```python
from build123d import *

# Parameters (mm, degrees)
SKETCH1_W              = 126
SKETCH1_H              = 126
BOSS_EXTRUDE1_DEPTH    = 5.5
CUT_EXTRUDE5_DEPTH     = 179.275769526
SKETCH8_R              = 10
CUT_EXTRUDE6_DEPTH     = 179.275769526
FILLET1_R              = 5.5
FILLET2_R              = 2.75
SKETCH11_W             = 13
SKETCH11_H             = 13
CUT_EXTRUDE7_DEPTH     = 179.275769526
BOSS_EXTRUDE8_START    = -15
SKETCH18_R             = 2
BOSS_EXTRUDE8_DEPTH    = 10
BOSS_EXTRUDE9_START    = -75
SKETCH18_2_R           = 2
BOSS_EXTRUDE9_DEPTH    = 10
BOSS_EXTRUDE10_DEPTH   = 10
BOSS_EXTRUDE11_DEPTH   = 3
BOSS_EXTRUDE12_DEPTH   = 4.692640137
BOSS_EXTRUDE12_START   = -13
BOSS_EXTRUDE12_2_DEPTH = 14
BOSS_EXTRUDE13_DEPTH   = 4.692640137
BOSS_EXTRUDE13_START   = -127
BOSS_EXTRUDE13_2_DEPTH = 14
CHAMFER1_SIZE          = 2


with BuildPart() as part:
    # Sketch1 → Boss-Extrude1 (new body)
    with BuildSketch(Plane(origin=(0, 0, 0), x_dir=(1, 0, 0), z_dir=(0, 1, 0))):
        with Locations((63, 63)):
            Rectangle(SKETCH1_W, SKETCH1_H)
    extrude(amount=BOSS_EXTRUDE1_DEPTH)

    # Sketch7 → Cut-Extrude5 (cut, through all)
    with BuildSketch(Plane.XY):
        Polygon((0, 0), (0, 5.5), (5.5, 5.5), align=None)
        Polygon((126, 0), (126, 5.5), (120.5, 5.5), align=None)
    cut_extrude5 = extrude(amount=-CUT_EXTRUDE5_DEPTH, mode=Mode.SUBTRACT)

    # Mirror1: Cut-Extrude5 across plane
    add(cut_extrude5.mirror(Plane(origin=(0, 0, 0), x_dir=(-0.7071067811865476, 0, 0.7071067811865476), z_dir=(-0.7071067811865477, 0, -0.7071067811865475))), mode=Mode.SUBTRACT)

    # Sketch8 → Cut-Extrude6 (cut, through all)
    with BuildSketch(Plane(origin=(0, 5.5, 0), x_dir=(1, 0, 0), z_dir=(0, 1, 0))):
        with Locations(Location((63, 63, 0), (0, 0, 270))):
            Circle(SKETCH8_R)
        with BuildLine():
            Line((50.269180349, 54.158267646), (8.5, 12.389087297))
            Line((8.5, 12.389087297), (8.5, 113.610912703))
            Line((8.5, 113.610912703), (50.269180349, 71.841732354))
            ThreePointArc((50.269180349, 71.841732354), (47.5, 63), (50.269180349, 54.158267646))
        make_face()
        with BuildLine():
            Line((54.158267646, 75.730819651), (12.389087297, 117.5))
            Line((12.389087297, 117.5), (113.610912703, 117.5))
            Line((113.610912703, 117.5), (71.841732354, 75.730819651))
            ThreePointArc((71.841732354, 75.730819651), (63, 78.5), (54.158267646, 75.730819651))
        make_face()
        with BuildLine():
            Line((75.730819651, 71.841732354), (117.5, 113.610912703))
            Line((117.5, 113.610912703), (117.5, 12.389087297))
            Line((117.5, 12.389087297), (75.730819651, 54.158267646))
            ThreePointArc((75.730819651, 54.158267646), (78.5, 63), (75.730819651, 71.841732354))
        make_face()
        with BuildLine():
            Line((71.841732354, 50.269180349), (113.610912703, 8.5))
            Line((113.610912703, 8.5), (12.389087297, 8.5))
            Line((12.389087297, 8.5), (54.158267646, 50.269180349))
            ThreePointArc((54.158267646, 50.269180349), (63, 47.5), (71.841732354, 50.269180349))
        make_face()
    extrude(amount=-CUT_EXTRUDE6_DEPTH, mode=Mode.SUBTRACT)

    # Fillet1
    fillet1_edges = [part.edges().sort_by_distance(p)[0] for p in [
        (113.610912703, 2.75, -8.5),
        (12.389087297, 2.75, -8.5),
        (117.5, 2.75, -113.610912703),
        (117.5, 2.75, -12.389087297),
        (12.389087297, 2.75, -117.5),
        (113.610912703, 2.75, -117.5),
        (8.5, 2.75, -12.389087297),
        (8.5, 2.75, -113.610912703),
    ]]
    fillet(fillet1_edges, radius=FILLET1_R)

    # Fillet2
    fillet2_edges = [part.edges().sort_by_distance(p)[0] for p in [
        (54.158267646, 2.75, -50.269180349),
        (71.841732354, 2.75, -50.269180349),
        (75.730819651, 2.75, -54.158267646),
        (75.730819651, 2.75, -71.841732354),
        (71.841732354, 2.75, -75.730819651),
        (54.158267646, 2.75, -75.730819651),
        (50.269180349, 2.75, -71.841732354),
        (50.269180349, 2.75, -54.158267646),
    ]]
    fillet(fillet2_edges, radius=FILLET2_R)

    # Sketch11 → Cut-Extrude7 (cut, through all)
    with BuildSketch(Plane(origin=(0, 5.5, 0), x_dir=(1, 0, 0), z_dir=(0, 1, 0))):
        with Locations((6.5, 119.5)):
            Rectangle(SKETCH11_W, SKETCH11_H)
        with Locations((119.5, 119.5)):
            Rectangle(SKETCH11_W, SKETCH11_H)
        with Locations((119.5, 6.5)):
            Rectangle(SKETCH11_W, SKETCH11_H)
        with Locations((6.5, 6.5)):
            Rectangle(SKETCH11_W, SKETCH11_H)
    extrude(amount=-CUT_EXTRUDE7_DEPTH, mode=Mode.SUBTRACT)

    # Sketch18 → Boss-Extrude8 (add)
    with BuildSketch(Plane(origin=(0, 0, -113), x_dir=(-1, 0, 0), z_dir=(0, 0, -1)).offset(BOSS_EXTRUDE8_START)):
        with BuildLine():
            Line((-6.5, 0), (0.5, 0))
            ThreePointArc((0.5, 0), (8.363703305, 1.03527618), (1.035898385, -2))
            Line((1.035898385, -2), (-6.5, -2))
            Line((-6.5, -2), (-6.5, 0))
        make_face()
        with Locations((4.5, 0)):
            Circle(SKETCH18_R, mode=Mode.SUBTRACT)
    extrude(amount=-BOSS_EXTRUDE8_DEPTH)

    # Sketch18<2> → Boss-Extrude9 (add)
    with BuildSketch(Plane(origin=(0, 0, -113), x_dir=(-1, 0, 0), z_dir=(0, 0, -1)).offset(BOSS_EXTRUDE9_START)):
        with BuildLine():
            Line((-6.5, 0), (0.5, 0))
            ThreePointArc((0.5, 0), (8.363703305, 1.03527618), (1.035898385, -2))
            Line((1.035898385, -2), (-6.5, -2))
            Line((-6.5, -2), (-6.5, 0))
        make_face()
        with Locations((4.5, 0)):
            Circle(SKETCH18_2_R, mode=Mode.SUBTRACT)
    extrude(amount=-BOSS_EXTRUDE9_DEPTH)

    # Sketch19 → Boss-Extrude10 (add)
    with BuildSketch(Plane.XZ):
        Polygon((126, -113), (113, -113), (113, -126), (110, -126), (110, -110), (126, -110), align=None)
        Polygon((126, -16), (126, -13), (113, -13), (113, 0), (110, 0), (110, -16), align=None)
    extrude(amount=BOSS_EXTRUDE10_DEPTH)

    # Sketch20 → Boss-Extrude11 (add)
    with BuildSketch(Plane.XZ.offset(10)):
        Polygon((110, -16), (126, -16), (126, -13), (128, -13), (128, 2), (113, 2), (113, 0), (110, 0), align=None)
        Polygon((126, -110), (126, -113), (128, -113), (128, -128), (113, -128), (113, -126), (110, -126), (110, -110), align=None)
    extrude(amount=BOSS_EXTRUDE11_DEPTH)

    # Boss-Extrude12: read off the stored shape, not the designer's step
    # Boss-Extrude12 outline → Boss-Extrude12 (add)
    with BuildSketch(Plane.ZY.offset(-13)):
        Polygon((-13, 5.5), (-13, 0), (0, 0), (-5.5, 5.5), align=None)
    extrude(amount=BOSS_EXTRUDE12_DEPTH)

    # Boss-Extrude12 2 outline → Boss-Extrude12 2 (cut)
    with BuildSketch(Plane.XY.offset(BOSS_EXTRUDE12_START)):
        with BuildLine():
            Line((8.307359863, 0), (11.819098493, 0))
            ThreePointArc((11.819098493, 0), (10.365939115, 2.943279669), (8.307359863, 5.5))
            Line((8.307359863, 5.5), (8.307359863, 0))
        make_face()
    extrude(amount=BOSS_EXTRUDE12_2_DEPTH, mode=Mode.SUBTRACT)

    # Boss-Extrude13: read off the stored shape, not the designer's step
    # Boss-Extrude13 outline → Boss-Extrude13 (add)
    with BuildSketch(Plane.ZY.offset(-13)):
        Polygon((-120.5, 5.5), (-126, 0), (-113, 0), (-113, 5.5), align=None)
    extrude(amount=BOSS_EXTRUDE13_DEPTH)

    # Boss-Extrude13 2 outline → Boss-Extrude13 2 (cut)
    with BuildSketch(Plane.XY.offset(BOSS_EXTRUDE13_START)):
        with BuildLine():
            ThreePointArc((11.819098492, 0), (10.365939114, 2.943279669), (8.307359863, 5.5))
            Line((8.307359863, 5.5), (8.307359863, 0))
            Line((8.307359863, 0), (11.819098492, 0))
        make_face()
    extrude(amount=BOSS_EXTRUDE13_2_DEPTH, mode=Mode.SUBTRACT)

    # Chamfer1
    chamfer1_edges = [part.edges().sort_by_distance(p)[0] for p in [
        (6.5, 0, -93),
        (6.5, 0, -33),
    ]]
    chamfer(chamfer1_edges, length=CHAMFER1_SIZE - 0.0001)  # a hair under: the kernel refuses the full size


solid = part.part
```
Verification items for the finished model (mm, model axes). A direction names the side the tool comes from. Give positions to 0.01 mm unless a question says otherwise; leave off trailing zeros. Loops run counter-clockwise (first coordinate to the right, second up) from the corner with the lowest first, then second, coordinate; pieces in that order, holes last.
1. Go/stop test with flat-tipped pins: pin 1 Ø0.6 at (y, z) = (-12, -127) entering from -X; pin 2 Ø8.5 at (x, z) = (3, -33.5) entering from -Y; pin 3 Ø4 at (x, z) = (2, -95.5) entering from -Y. Record where each tip stops, or that it passes through.
2. Set-up check for faces 5 (the cylindrical face through (11.81, 2.71, -20.62)), 6 (the flat face through (113, -2, -6)), 7 (the flat face through (3, -2, -93)), 8 (the flat face through (118, -6, -16)): record each of +Z, -Z, +X, -X, +Y, -Y from which the full face is reachable in a straight line by a thin tool's end or side.
3. Section check C-C, the plane x = 63. Enter the section's corners in (y, z).
4. Thickness scan on line 1 (Z direction, x = 115.5, y = -1.25); line 2 (X direction, y = 3.5, z = -69); line 3 (X direction, y = 1.25, z = -96). Record the ranges inside material, lowest first.
5. Section check A-A, the plane y = -5.75. Enter the section's corners in (x, z), then the cut area to 3 significant figures.
6. Section check B-B, the plane z = -63. Enter the section's corners in (x, y).
7. Mould release check, pull along X, two halves, no side actions. Record for faces 1 (the cylindrical face through (57, 3, -71)), 2 (the flat face through (88.57, 2.79, -33.54)), 3 (the flat face through (120, -10, -5)), 4 (the flat face through (123, 3, -62)): released by +X, released by -X, zero draft, split by the parting line, or undercut.
Geometry says:
1. pin 1: stops at x = 113
1. pin 2: stops at y = -2.33
1. pin 3: stops at y = -2
2. face 5: +Y, -Y
2. face 6: +Z, +X, +Y
2. face 7: +Z, -Z, +X, -Y
2. face 8: +X, -X, -Y
3. outline: (0, -126) - (5.5, -120.5) - (5.5, -117.5) - (0, -117.5) - close; (0, -78.5) - (5.5, -78.5) - (5.5, -73) - (0, -73) - close; (0, -53) - (5.5, -53) - (5.5, -47.5) - (0, -47.5) - close; (0, -8.5) - (5.5, -8.5) - (5.5, -5.5) - (0, 0) - close
4. line 1: z = -113 to -110, -16 to -13
4. line 2: x = 3.5 to 8.5, 48.71 to 55, 71 to 77.29, 117.5 to 122.5
4. line 3: x = -8.3 to -6.06, -2.94 to -0.7, 1.25 to 8.5, 26.11 to 33.89, 92.11 to 99.89, 117.5 to 124.75
5. outline: (110, -126) - (113, -126) - (113, -113) - (126, -113) - (126, -110) - (110, -110) - close; (110, -16) - (126, -16) - (126, -13) - (113, -13) - (113, 0) - (110, 0) - close
5. area: 174 mm2
6. outline: (0, 0) - (8.5, 0) - (8.5, 5.5) - (5.5, 5.5) - close; (47.5, 0) - (53, 0) - (53, 5.5) - (47.5, 5.5) - close; (73, 0) - (78.5, 0) - (78.5, 5.5) - (73, 5.5) - close; (117.5, 0) - (126, 0) - (120.5, 5.5) - (117.5, 5.5) - close
7. face 1: undercut
7. face 2: undercut
7. face 3: zero draft
7. face 4: released by +X
